Build history of the part. All positions in model axes, mm. Face numbers are marked on the shaded views. A direction names the side the tool comes from. Give positions to 0.01 mm unless a question says otherwise; leave off trailing zeros. Order: outer loops, then holes, each group sorted by start corner. A loop starts at its lowest first (then second) coordinate and runs counter-clockwise, first axis right, second up. Notation, with made-up numbers: M 65.25,40.25 L 84.25,40.25 A15 cw 84.25,66.25 Z; hole C -26.5,-36 d10. An arc over 180 degrees is marked long. One line per item, written item: value.
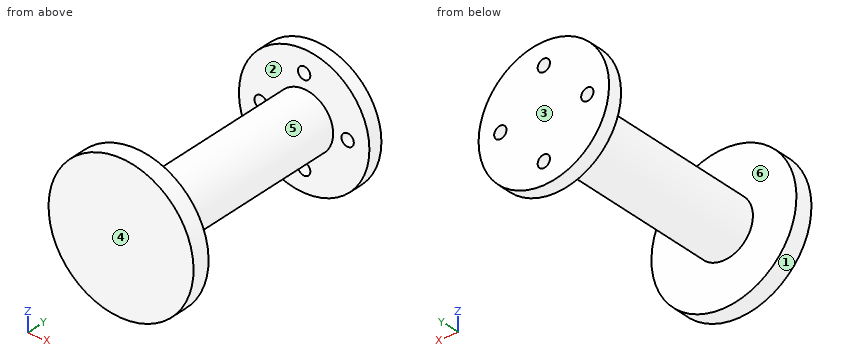
from build123d import *

# Parameters (mm, degrees)
SKETCH_2_R          = 1.7
CUT_EXTRUDE_1_DEPTH = 10


with BuildPart() as part:
    # 草图1 → 旋转1 (revolve)
    with BuildSketch(Plane.XY, mode=Mode.PRIVATE) as revolve_1_sk:
        Polygon((0, 0), (-20, 0), (-20, 5), (-8, 5), (-8, 61), (-18, 61), (-18, 65), (0, 65), align=None)
    revolve(revolve_1_sk.sketch.rotate(Axis((0, 0, 0), (0, 1, 0)), 270), axis=Axis((0, 0, 0), (0, 1, 0)))

    # 草图2 → 切除-拉伸1 (cut)
    with BuildSketch(Plane(origin=(0, 65, 0), x_dir=(1, 0, 0), z_dir=(0, 1, 0))):
        with Locations(Location((12, 0, 0), (0, 0, 270))):
            Circle(SKETCH_2_R)
        with Locations(Location((0, -12, 0), (0, 0, 270))):
            Circle(SKETCH_2_R)
        with Locations(Location((-12, 0, 0), (0, 0, 270))):
            Circle(SKETCH_2_R)
        with Locations(Location((0, 12, 0), (0, 0, 270))):
            Circle(SKETCH_2_R)
    extrude(amount=-CUT_EXTRUDE_1_DEPTH, mode=Mode.SUBTRACT)


solid = part.part
1) Saw through at B-B, the plane x = -17. Write the cut outline in (y, z).
Check values:
outline: M 0,-10.54 L 5,-10.54 L 5,10.54 L 0,10.54 Z; M 61,-5.92 L 65,-5.92 L 65,5.92 L 61,5.92 Z
2) Saw through at C-C, the plane x = -12. Write the cut outline in (y, z), then the cut area to 3 significant figures.
Check values:
outline: M 0,-16 L 5,-16 L 5,16 L 0,16 Z; M 61,-13.42 L 65,-13.42 L 65,-1.7 L 61,-1.7 Z; M 61,1.7 L 65,1.7 L 65,13.42 L 61,13.42 Z
area: 254 mm^2
3) Mould opens along Y. For the marked faces 3, 4, 5 and 6 say: released by +Y, released by -Y, zero draft, split by the parting line, or undercut.
Check values:
face 3: released by +Y
face 4: released by -Y
face 5: undercut
face 6: undercut
4) Saw through at A-A, the plane z = 15.5. Write the cut outline in (x, y), then the cut area to 3 significant figures.
Check values:
outline: M -12.64,0 L 12.64,0 L 12.64,5 L -12.64,5 Z; M -9.15,61 L 9.15,61 L 9.15,65 L -9.15,65 Z
area: 200 mm^2
5) Drill centre lines: probe 1 along X at (y, z) = (62.6, 0); probe 2 along Y at (x, z) = (1, 14.5); probe 3 along Y at (x, z) = (11, -15.5). Where is each one in solid material? Low to high. Write a range as from..to.
Check values:
probe 1: -18..-13.7, -10.3..10.3, 13.7..18
probe 2: 0..5, 61..65
probe 3: 0..5
6) Saw through at D-D, the plane z = -5. Write the cut outline in (x, y) (3 decimals), then the cut area to 3 significant figures.
Check values:
outline: M -19.365,0 L 19.365,0 L 19.365,5 L 6.245,5 L 6.245,61 L 17.292,61 L 17.292,65 L -17.292,65 L -17.292,61 L -6.245,61 L -6.245,5 L -19.365,5 Z
area: 1,030 mm^2
7) Pin check, flat tips, straight feed: pin 1 (6 mm diameter, centred on x = 9.5, y = 31, fed in from -Z); pin 2 (2.5 mm diameter, centred on x = 12, z = 0, fed in from +Y); pin 3 (2 mm diameter, centred on x = -2, y = 27.5, fed in from -Z); pin 4 (4 mm diameter, centred on x = 0, z = 12, fed in from -Y). Stop position of each tip, or through.
Check values:
pin 1: z = -4.66
pin 2: y = 5
pin 3: z = -7.94
pin 4: y = 0
8) Tool access for the marked faces 1 and 2: list every direction of +Z, -Z, +X, -X, +Y, -Y with a clear straight run to the whole face (end or side of a thin tool).
Check values:
face 1: +Y, -Y
face 2: none
